from build123d import *

# Parameters (mm, degrees)
SKETCH2_R            = 12.7
BOSS_EXTRUDE1_DEPTH  = 12.7
BOSS_EXTRUDE2_DEPTH  = 6.35
CUT_EXTRUDE1_START   = -6.35
CUT_EXTRUDE1_DEPTH   = 7.62
BOSS_EXTRUDE3_DEPTH  = 6.35
SKETCH6_R            = 3.81
BOSS_EXTRUDE4_DEPTH  = 12.7
BOSS_EXTRUDE5_START  = -1.27
SKETCH7_R            = 7.64274541
SKETCH7_R_2          = 3.81
BOSS_EXTRUDE5_DEPTH  = 5.08
CUT_EXTRUDE2_DEPTH   = 94.001963864
SKETCH14_R           = 7.62
CUT_EXTRUDE3_DEPTH   = 6.35
BOSS_EXTRUDE12_REACH = 93.815
FILLET1_R            = 2.54
CUT_EXTRUDE5_REACH   = 105.401
SKETCH16_W           = 3.81
SKETCH16_H           = 8.99772588


with BuildPart() as part:
    # Sketch2 → Boss-Extrude1 (new body)
    with BuildSketch(Plane(origin=(0, 0, 0), x_dir=(1, 0, 0), z_dir=(0, 1, 0))):
        with Locations(Location((0, 0, 0), (0, 0, 270))):
            Circle(SKETCH2_R)
    extrude(amount=BOSS_EXTRUDE1_DEPTH)

    # Sketch3 → Boss-Extrude2 (add, symmetric)
    with BuildSketch(Plane.XY):
        with BuildLine():
            Line((6.35, 12.7), (-28.263014494, 50.680235189))
            ThreePointArc((-28.263014494, 50.680235189), (-36.606963582, 54.691505771), (-34.105544768, 45.777770191))
            Line((-34.105544768, 45.777770191), (-6.35, 12.7))
            Line((-6.35, 12.7), (6.35, 12.7))
        make_face()
    extrude(amount=BOSS_EXTRUDE2_DEPTH, both=True)

    # Sketch4 → Cut-Extrude1 (cut, symmetric)
    with BuildSketch(Plane.XY.offset(6.35).offset(CUT_EXTRUDE1_START)):
        with BuildLine():
            Line((-5.757789274, 13.97), (3.474314319, 13.97))
            Line((3.474314319, 13.97), (-29.573983747, 50.233300134))
            ThreePointArc((-29.573983747, 50.233300134), (-35.779559637, 53.727877238), (-33.46657952, 46.992050322))
            Line((-33.46657952, 46.992050322), (-5.757789274, 13.97))
        make_face()
    extrude(amount=CUT_EXTRUDE1_DEPTH, both=True, mode=Mode.SUBTRACT)

    # Sketch5 → Boss-Extrude3 (add, symmetric)
    with BuildSketch(Plane.XY):
        Polygon((-23.82267484, 43.922492823), (-20.27066661, 40.024938393), (-30.298747694, 43.216775363), (-33.46657952, 46.992050322), align=None)
        Polygon((-20.27066661, 40.024938393), (-20.27066661, 31.265773704), (-17.73066661, 28.238719579), (-17.73066661, 37.237842303), align=None)
        Polygon((-5.458773455, 23.772115752), (-1.772739842, 19.727497693), (-14.465305553, 24.347213808), (-17.73066661, 28.238719579), align=None)
    extrude(amount=BOSS_EXTRUDE3_DEPTH, both=True)

    # Sketch6 → Boss-Extrude4 (add, symmetric)
    with BuildSketch(Plane.XY):
        with Locations((-33.341602525, 50.8)):
            Circle(SKETCH6_R)
    extrude(amount=BOSS_EXTRUDE4_DEPTH, both=True)

    # Sketch7 → Boss-Extrude5 (add)
    # profile 1 of 4: a face of its own
    with BuildSketch(Plane.XY.offset(12.7).offset(BOSS_EXTRUDE5_START)):
        with Locations((-33.341602525, 50.8)):
            Circle(SKETCH7_R)
        with Locations(Location((-33.341602525, 50.8, 0), (0, 0, 268.120225958))):
            Circle(SKETCH7_R_2, mode=Mode.SUBTRACT)
    # profile 2 of 4: a face of its own
    with BuildSketch(Plane.XY.offset(12.7).offset(BOSS_EXTRUDE5_START)):
        with BuildLine():
            ThreePointArc((-28.428940471, 44.945317348), (-38.558455358, 45.2146617), (-39.517448502, 55.302275411))
            Line((-39.517448502, 55.302275411), (-66.450706217, 18.357478363))
            Line((-66.450706217, 18.357478363), (-61.506739525, 17.189748362))
            Line((-61.506739525, 17.189748362), (-28.428940471, 44.945317348))
        make_face()
    # profile 3 of 4: a face of its own
    with BuildSketch(Plane.XY.offset(12.7).offset(BOSS_EXTRUDE5_START)):
        Polygon((-61.506739525, 17.189748362), (-63.258334527, 9.773798325), (-68.202301218, 10.941528326), (-66.450706217, 18.357478363), align=None)
    # profile 4 of 4: a face of its own
    with BuildSketch(Plane.XY.offset(12.7).offset(BOSS_EXTRUDE5_START)):
        Polygon((-68.202301218, 10.941528326), (-63.258334527, 3.423798325), (-63.258334527, 9.773798325), align=None)
    extrude(amount=-BOSS_EXTRUDE5_DEPTH)

    # Sketch10 → Cut-Extrude2 (cut, through all)
    with BuildSketch(Plane.XY.offset(11.43)):
        Polygon((-43.431264654, 47.562180038), (-51.48051274, 36.520892717), (-40.182838097, 36.906280169), align=None)
        Polygon((-52.976804835, 34.468403992), (-53.949591662, 25.35460233), (-42.669146252, 34.820019913), align=None)
        Polygon((-55.05214832, 31.621620856), (-61.893965932, 22.236585976), (-55.895344547, 23.721921802), align=None)
        Polygon((-64.655334527, 9.936540168), (-65.75979615, 15.205273966), (-66.70434579, 11.206214291), (-64.655334527, 8.090515014), align=None)
        Polygon((-63.390258027, 20.184097251), (-65.155875161, 17.762170896), (-64.051413538, 12.493437098), (-62.759783939, 17.96197324), (-58.739005045, 21.335807327), align=None)
        Polygon((-41.708282924, 49.925622701), (-38.237085212, 38.538960697), (-33.643800576, 42.393184141), align=None)
    extrude(amount=-CUT_EXTRUDE2_DEPTH, mode=Mode.SUBTRACT)

    # Mirror1: part across plane


with BuildPart() as part_1:
    add(part.part)
    add(part.part.mirror(Plane.XY))

    # Sketch14 → Cut-Extrude3 (cut)
    with BuildSketch(Plane.XZ):
        with Locations(Location((0, 0, 0), (0, 0, 270))):
            Circle(SKETCH14_R)
    extrude(amount=-CUT_EXTRUDE3_DEPTH, mode=Mode.SUBTRACT)

    # Sketch15 → Boss-Extrude12 (add, up to next)
    with BuildSketch(Plane.XY.offset(-6.35), mode=Mode.PRIVATE) as boss_extrude12_sk1:
        Polygon((-64.9758417, 18.009125785), (-66.450706217, 18.357478363), (-68.202301218, 10.941528326), (-63.258334527, 3.423798325), (-63.258334527, 9.773798325), (-61.506739525, 17.189748362), (-62.866330365, 17.510874112), (-64.051413538, 12.493437098), (-65.155875161, 17.762170896), align=None)
        Polygon((-64.655334527, 8.090515014), (-66.70434579, 11.206214291), (-65.75979615, 15.205273966), (-64.655334527, 9.936540168), align=None, mode=Mode.SUBTRACT)
    boss_extrude12_tool1 = extrude(boss_extrude12_sk1.sketch, amount=BOSS_EXTRUDE12_REACH, mode=Mode.PRIVATE) - part_1.part
    add(boss_extrude12_tool1.solids().sort_by_distance((-64.87727, 11.921902, -6.35))[0])

    # Fillet1
    fillet1_edges = [part_1.edges().sort_by_distance(p)[0] for p in [
        (0, 0, -12.7),
        (0, 12.7, -12.7),
    ]]
    fillet(fillet1_edges, radius=FILLET1_R)

    # Sketch16 → Cut-Extrude5 (cut, up to next)
    with BuildSketch(Plane(origin=(-42.587828759, -28.007497849, 0), x_dir=(0, 0, 1), z_dir=(-0.835514451237255, -0.54946847204704, 0)), mode=Mode.PRIVATE) as cut_extrude5_sk1:
        with Locations((-4.445, 42.117956336)):
            Rectangle(SKETCH16_W, SKETCH16_H)
    cut_extrude5_tool1 = extrude(cut_extrude5_sk1.sketch, amount=-CUT_EXTRUDE5_REACH, mode=Mode.PRIVATE) & part_1.part
    # Sketch16 → Cut-Extrude5 (cut, up to next)
    with BuildSketch(Plane(origin=(-42.587828759, -28.007497849, 0), x_dir=(0, 0, 1), z_dir=(-0.835514451237255, -0.54946847204704, 0)), mode=Mode.PRIVATE) as cut_extrude5_sk2:
        with Locations((4.445, 42.117956336)):
            Rectangle(SKETCH16_W, SKETCH16_H)
    cut_extrude5_tool2 = extrude(cut_extrude5_sk2.sketch, amount=-CUT_EXTRUDE5_REACH, mode=Mode.PRIVATE) & part_1.part
    add(cut_extrude5_tool1.solids().sort_by_distance((-65.730318, 7.182663, -4.445))[0], mode=Mode.SUBTRACT)
    add(cut_extrude5_tool2.solids().sort_by_distance((-65.730318, 7.182663, 4.445))[0], mode=Mode.SUBTRACT)


solid = part_1.part
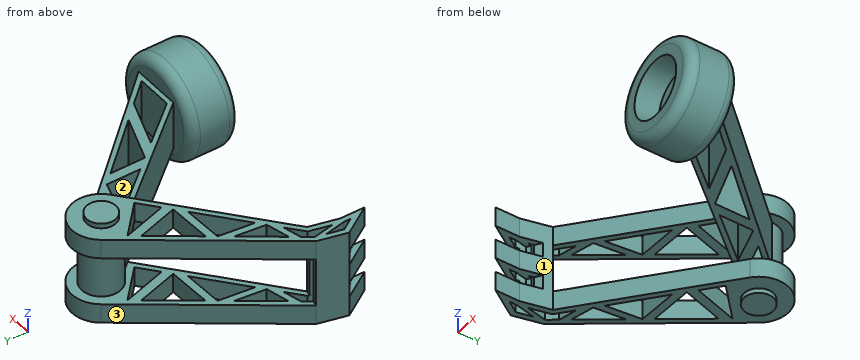
Build history of the part. All positions in model axes, mm. Face numbers are marked on the shaded views. A direction names the side the tool comes from. Coordinates: 2 decimals unless noted, no trailing zeros. Order: outer loops, then holes, each group sorted by start corner. A loop starts at its lowest first (then second) coordinate and runs counter-clockwise, first axis right, second up. Notation, with made-up numbers: (0.25, -5.5) - (7.25, -5.5) arc R15 ccw to (7.25, 11.5) - close; hole circle Ø8 at (58, -17). An arc over 180 degrees is marked (long way). Write item = value, one per line. Start each with the question number.
1) Saw through at C-C on z = 0. Count the separate pieces of the cut face and the enclosed holes in it, then the cut area to 3 significant figures.
2) Saw through at D-D on x = -47. Write the cut outline in (y, z), then the cut area to 3 significant figures.
3) Saw through at A-A on y = 4.5. Write the cut outline in (x, z).
4) 3-axis set-ups, long thin cutter, end or side, ignore diameter. For the marked faces 1, 2 and 3: which of +Z, -Z, +X, -X, +Y, -Y reach the whole face in a straight line?
5) Flat gauge pins, fed straight in: pin 1 Ø2.5 at (y, z) = (38, 1) entering from -X; pin 2 Ø1 at (x, y) = (-43, 48.5) entering from +Z; pin 3 Ø2.5 at (y, z) = (33, 2) entering from +X. Where does each tip first touch, or does it go through?
6) Wall check: line 1 along Y through (x, z) = (-48, -11.25); line 2 along X through (y, z) = (3.75, 0); line 3 along Y through (x, z) = (-50, 10). Give the ranges that are in metal, low to high. Write a range as from..to.
7) Saw through at B-B on x = 0. Write the cut outline in (y, z), then the cut area to 3 significant figures.
From the geometry:
q1.separate_pieces = 2
q1.enclosed_holes = 5
q1.area = 550 mm^2
q2.outline = (29.36, -11.43) - (31.19, -11.43) - (31.19, -6.35) - (29.36, -6.35) - close; (29.36, 6.35) - (31.19, 6.35) - (31.19, 11.43) - (29.36, 11.43) - close; (34.67, -11.43) - (36.67, -11.43) - (36.67, -6.35) - (34.67, -6.35) - close; (34.67, 6.35) - (36.67, 6.35) - (36.67, 11.43) - (34.67, 11.43) - close; (42.67, -11.43) - (45.04, -11.43) - (45.04, -6.35) - (42.67, -6.35) - close; (42.67, 6.35) - (45.04, 6.35) - (45.04, 11.43) - (42.67, 11.43) - close
q2.area = 63.0 mm^2
q3.outline = (-63.97, -11.43) - (-63.26, -11.43) - (-63.26, -6.35) - (-63.97, -6.35) - close; (-63.97, -2.54) - (-63.26, -2.54) - (-63.26, 2.54) - (-63.97, 2.54) - close; (-63.97, 6.35) - (-63.26, 6.35) - (-63.26, 11.43) - (-63.97, 11.43) - close; circle Ø25.4 at (0, 0); hole circle Ø15.24 at (0, 0)
q4.face_1 = +Z, -Z, -Y
q4.face_2 = +Z, -Z
q4.face_3 = +Z, -Z, -X, +Y
q5.pin_1 = -28.63
q5.pin_2 = 11.43
q5.pin_3 = -11.01
q6.line_1 = 28.52..30.35, 34.64..36.64, 41.3..43.67
q6.line_2 = -63.47..-63.26, -12.7..-7.62, 7.62..12.7
q6.line_3 = 26.85..28.67, 34.57..36.57, 38.55..40.92
q7.outline = (0, -10.16) arc R2.54 ccw to (2.54, -12.7) - (10.16, -12.7) arc R2.54 ccw to (12.7, -10.16) - (12.7, -6.35) - (13.97, -6.35) - (13.97, 6.35) - (12.7, 6.35) - (12.7, 10.16) arc R2.54 ccw to (10.16, 12.7) - (2.54, 12.7) arc R2.54 ccw to (0, 10.16) - (0, 7.62) - (6.35, 7.62) - (6.35, -7.62) - (0, -7.62) - close; (17.78, -6.35) - (19.67, -6.35) - (19.67, 6.35) - (17.78, 6.35) - close
q7.area = 260 mm^2
